Geometry: see drawing. Coordinates: mm, zero at the bounding-box minimum. A direction names the side the tool comes from. Round coordinates to 2 decimals unless told otherwise and drop trailing zeros. Loops run counter-clockwise (first coordinate to the right, second up) from the corner with the lowest first, then second, coordinate; pieces in that order, holes last. Notation, with made-up numbers: (-35, -27.75) - (16, -27.75) arc R25 cw to (16, 5.25) - close; hole circle Ø5 at (23.5, -7). An arc over 180 degrees is marked (long way). Use CSV: the item, a comma, the result in double quotes. Start each with the question number.
1. Cut plane C-C (y = 5.35). Return loops of the section in (x, z) (1 decimal), and give its area (3 significant figures).
2. Material intervals for probe 1 along Y at (x, z) = (3, 4.8); probe 2 along Y at (x, z) = (3.65, 18.25); probe 3 along X at (y, z) = (2.4, 1) (1 decimal), sorted ascending. Write a range as from..to.
3. Cut plane A-A (z = 15.25). Return loops of the section in (x, y).
4. Pin query (flat end, axial travel): P1, Ø1, axis at x = 5.5, z = 11, coming from the +Y side (1 decimal); P2, Ø2.5, axis at x = 3, y = 3, coming from the -Z side; P3, Ø1.5, axis at x = 5.5, z = 8, coming from the +Y side. Return the tip coordinate at first contact, or that it passes through.
5. Access query for the marked faces 4 and 5. Directions: +Z, -Z, +X, -X, +Y, -Y. A direction counts if a zero-diameter tool reaches every point of the face in a straight line with its end or side. Return the directions, or none.
6. Pull-direction query (X, two-part tool) for the marked faces 1, 2 and 3; classes: +X half, -X half, draft (parallel to the pull), parting line (faces both ways), or undercut.
7. Cut plane B-B (x = 0.6). Return loops of the section in (y, z).
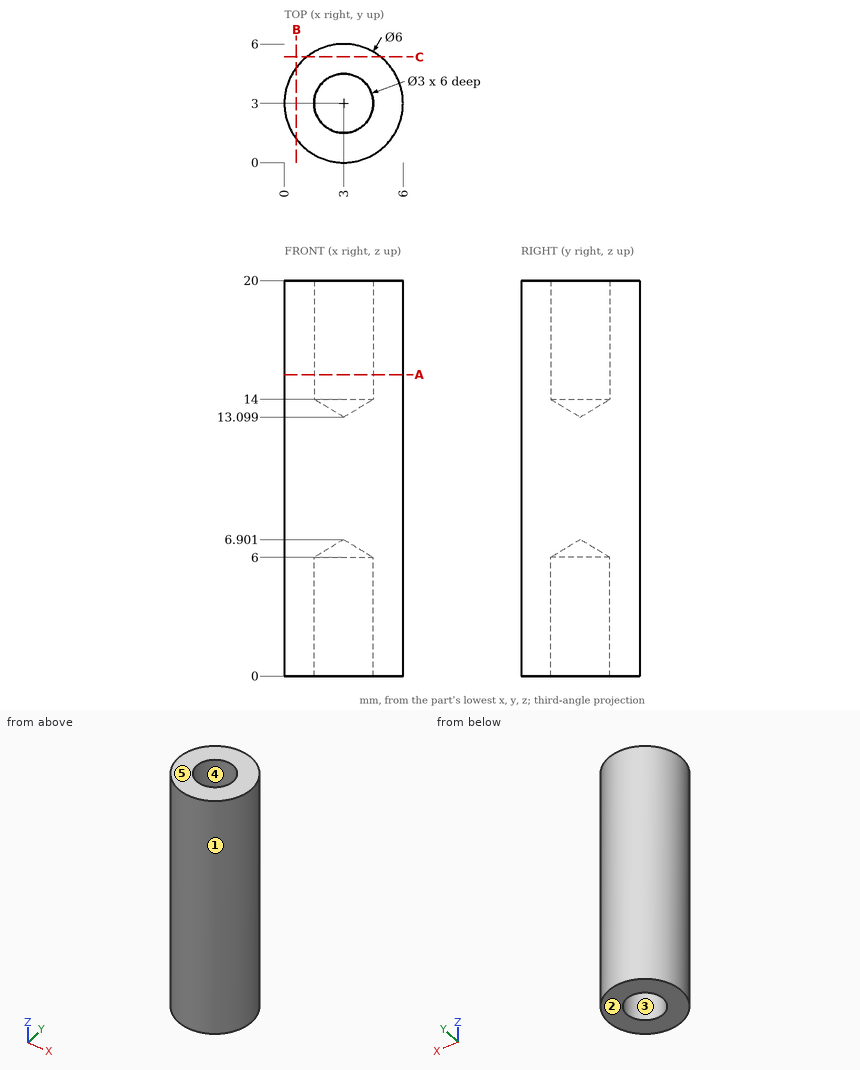
Established:
1,outline,"(1.1, 0) - (4.9, 0) - (4.9, 20) - (1.1, 20) - close"
1,area,"74.6 mm2"
2,probe 1,"y = 0..1.5, 4.5..6"
2,probe 2,"y = 0.07..1.65, 4.35..5.93"
2,probe 3,"x = 0.1..1.6, 4.4..5.9"
3,outline,"circle Ø6 at (3, 3); hole circle Ø3 at (3, 3)"
4,P1,"stops at y = 5.2"
4,P2,"stops at z = 6.15"
4,P3,"stops at y = 5.44"
5,face 4,"+Z"
5,face 5,"+Z, +X, -X, +Y, -Y"
6,face 1,"parting line"
6,face 2,"draft"
6,face 3,"undercut"
7,outline,"(1.2, 0) - (4.8, 0) - (4.8, 20) - (1.2, 20) - close"
